Can you work these out from the model? Positions are in its coordinate system, mm. A direction names the side the tool comes from. Give positions to 0.01 mm unless a question says otherwise; leave off trailing zeros. Order: outer loops, then holes, each group sorted by start corner. A loop starts at its lowest first (then second) coordinate and runs counter-clockwise, first axis right, second up. Notation, with made-up numbers: M 12.5,42 L 58.5,42 A9 cw 58.5,57 Z; hole C 39,-38 d4. An arc over 180 degrees is marked long. Use one line per item in the form item = value. Start each with the question number.
1. We'd pull the mould along X, two halves only. Please class faces 1 (the face through (39, 26, 150)), 2 (the face through (102.63, 72, 22)), 3 (the face through (104.63, 48, 76)), 4 (the face through (102.63, 23, 22)): +X half, -X half, draft (parallel to the pull), parting line (faces both ways), or undercut.
2. Will these pins go through, and if not, where does the flat tip stop? P1, Ø12, axis at x = 46, y = 27.5, coming from the -Z side; P2, Ø0.6, axis at x = 103.5, z = 29, coming from the -Y side; P3, Ø1.6, axis at x = -1, z = 151.5, coming from the -Y side; P4, Ø15, axis at x = 73, y = 8.5, coming from the -Z side.
3. I want a section at C-C, the plane x = 39.5. List the corners of the cut face in (y, z) for me.
4. I want a section at A-A, the plane y = 63. List the corners of the cut face in (x, z) for me, and give its area (3 significant figures).
5. I want a section at D-D, the plane x = 51.5. List the corners of the cut face in (y, z) for me.
6. I need wall thicknesses on L1, parallel to X at y = 40, z = 111.5; L2, parallel to Z at x = 46, y = 15; L3, parallel to Y at x = 34, z = 92. Which ranges of each line are inside material? Lowest first, please.
7. For faces 5 (the face through (48.034, 89.376, 0.986)), 6 (the face through (39, 77, 149)), 7 (the face through (-2, 48, 76)), which set-ups out of +Z, -Z, +X, -X, +Y, -Y let a thin tool reach every point of the face, with its end or its side?
8. I want a section at B-B, the plane z = 29. List the corners of the cut face in (x, y) for me, and give its area (3 significant figures).
```python
from build123d import *

# Parameters (mm, degrees)
BOSS_EXTRUDE1_DEPTH   = 150
BOSS_EXTRUDE3_DEPTH   = 1
BOSS_EXTRUDE3_2_DEPTH = 1
BOSS_EXTRUDE5_DEPTH   = 2
BOSS_EXTRUDE6_DEPTH   = 2
SKETCH8_W             = 40
SKETCH8_H             = 5
BOSS_EXTRUDE7_DEPTH   = 2


with BuildPart() as part:
    # Sketch1 → Boss-Extrude1 (new body)
    with BuildSketch(Plane.XY):
        Polygon((104.63, 25.965351431), (104.63, 69.034648569), (-2, 97.60645993), (-2, -2.60645993), align=None)
        Polygon((102.63, 67.5), (0, 95), (0, 0), (102.63, 27.5), align=None, mode=Mode.SUBTRACT)
    extrude(amount=BOSS_EXTRUDE1_DEPTH)



with BuildPart() as body_2:
    # Sketch3 → Boss-Extrude3 (new body)
    with BuildSketch(Plane.XY.offset(150)):
        Polygon((0, 65.5), (102.63, 65.5), (102.63, 67.5), (0, 95), align=None)
    extrude(amount=-BOSS_EXTRUDE3_DEPTH)


with BuildPart() as body_3:
    # Sketch3 → Boss-Extrude3 2 (new body)
    with BuildSketch(Plane.XY.offset(150)):
        Polygon((102.63, 27.5), (102.63, 29.5), (0, 29.5), (0, 0), align=None)
    extrude(amount=-BOSS_EXTRUDE3_2_DEPTH)


with BuildPart() as part_1:
    add(part.part)

    add(body_2.part)  # Boss-Extrude5 merges body 2

    add(body_3.part)  # Boss-Extrude5 merges body 3
    # Sketch6 → Boss-Extrude5 (add)
    with BuildSketch(Plane.ZY.offset(2)):
        Polygon((150, 67.5), (151.5, 67.5), (151.5, 27.5), (150, 27.5), (150, -2.60645993), (153, -2.60645993), (153, 97.60645993), (150, 97.60645993), align=None)
    extrude(amount=-BOSS_EXTRUDE5_DEPTH)

    # Sketch7 → Boss-Extrude6 (add)
    with BuildSketch(Plane(origin=(0, 0, 0), x_dir=(-1, 0, 0), z_dir=(0, 0, -1))):
        Polygon((-104.63, 20.788965809), (7, -9.122609754), (7, 104.122609754), (-104.63, 74.211034191), (-104.63, 69.034648569), (2, 97.60645993), (2, -2.60645993), (-104.63, 25.965351431), align=None)
    extrude(amount=-BOSS_EXTRUDE6_DEPTH)

    # Sketch8 → Boss-Extrude7 (add)
    with BuildSketch(Plane(origin=(104.63, 0, 0), x_dir=(0, 0, -1), z_dir=(1, 0, 0))):
        with Locations((-22, 71.534648569)):
            Rectangle(SKETCH8_W, SKETCH8_H)
        with Locations((-22, 23.465351431)):
            Rectangle(SKETCH8_W, SKETCH8_H)
    extrude(amount=-BOSS_EXTRUDE7_DEPTH)


solid = part_1.part
```
Check result:
q1.face_1 = draft
q1.face_2 = undercut
q1.face_3 = +X half
q1.face_4 = undercut
q2.P1 = 149
q2.P2 = 20.97
q2.P3 = -2.61
q2.P4 = 0
q3.outline = M 3.34,0 L 10.58,0 L 10.58,149 L 29.5,149 L 29.5,150 L 8.51,150 L 8.51,2 L 3.34,2 Z; M 65.5,149 L 84.42,149 L 84.42,0 L 91.66,0 L 91.66,2 L 86.49,2 L 86.49,150 L 65.5,150 Z
q4.outline = M -7,0 L 0,0 L 0,150 L -2,150 L -2,2 L -7,2 Z; M -2,151.5 L 0,151.5 L 0,153 L -2,153 Z; M 102.63,0 L 104.63,0 L 104.63,150 L 102.63,150 Z
q4.area = 613 mm2
q5.outline = M 6.55,0 L 13.8,0 L 13.8,149 L 29.5,149 L 29.5,150 L 11.73,150 L 11.73,2 L 6.55,2 Z; M 65.5,149 L 81.2,149 L 81.2,0 L 88.45,0 L 88.45,2 L 83.27,2 L 83.27,150 L 65.5,150 Z
q6.L1 = -2 to 0, 102.63 to 104.63
q6.L2 = 149 to 150
q6.L3 = 7.04 to 9.11, 85.89 to 87.96
q7.face_5 = +Z, -Z, +X, +Y
q7.face_6 = -Z
q7.face_7 = +Z, -X, +Y, -Y
q8.outline = M -2,-2.61 L 102.63,25.43 L 102.63,20.97 L 104.63,20.97 L 104.63,74.03 L 102.63,74.03 L 102.63,69.57 L -2,97.61 Z; hole M 0,0 L 102.63,27.5 L 102.63,67.5 L 0,95 Z
q8.area = 730 mm2
